Design review of the part built by this model. Coordinates are the model's own, in mm. Give positions to 0.01 mm unless a question says otherwise; leave off trailing zeros. Write each loop counter-clockwise with the first axis right and the second up, starting at its lowest first coordinate (ties: lowest second). Pieces come first, ordered by that corner, then holes. Notation, with made-up numbers: (-3, -5.75) -> (48, -5.75) arc R17 ccw to (48, 21.25) -> close; hole circle Ø10 at (88.25, 19). An arc over 180 degrees is marked (long way). Answer as a JSON object with one key per item and string values.
```python
from build123d import *

# Parameters (mm, degrees)
SKETCH1_W                        = 35
SKETCH1_H                        = 42.3
SKETCH1_W_2                      = 42.3
BOSS_EXTRUDE1_DEPTH              = 2
F_1_8_0_125_DIAMETER_HOLE1_D     = 3.175
F_1_8_0_125_DIAMETER_HOLE1_DEPTH = 4.5
F_1_8_0_125_DIAMETER_HOLE1_TIP   = 0.953866233
SKETCH4_R                        = 11.5
CUT_EXTRUDE1_DEPTH               = 2
CHAMFER1_SIZE                    = 5


with BuildPart() as part:
    # Sketch1 → Boss-Extrude1 (new body)
    with BuildSketch(Plane.XY):
        with Locations((-38.65, 0)):
            Rectangle(SKETCH1_W, SKETCH1_H)
        Rectangle(SKETCH1_W_2, SKETCH1_H)
    extrude(amount=BOSS_EXTRUDE1_DEPTH)

    # 1/8 (0.125) Diameter Hole1
    with Locations(Plane.XY.offset(2)):
        with Locations((-15.5, 15.5), (15.5, 15.5), (15.5, -15.5), (-15.5, -15.5)):
            Hole(F_1_8_0_125_DIAMETER_HOLE1_D / 2, depth=F_1_8_0_125_DIAMETER_HOLE1_DEPTH)
            with Locations((0, 0, -(F_1_8_0_125_DIAMETER_HOLE1_DEPTH + F_1_8_0_125_DIAMETER_HOLE1_TIP / 2))):  # 118° drill point
                Cone(0, F_1_8_0_125_DIAMETER_HOLE1_D / 2, F_1_8_0_125_DIAMETER_HOLE1_TIP, mode=Mode.SUBTRACT)

    # Sketch4 → Cut-Extrude1 (cut)
    with BuildSketch(Plane.XY.offset(2)):
        Circle(SKETCH4_R)
    extrude(amount=-CUT_EXTRUDE1_DEPTH, mode=Mode.SUBTRACT)

    # Chamfer1
    chamfer1_edges = [part.edges().sort_by_distance(p)[0] for p in [
        (21.15, 21.15, 1),
        (21.15, -21.15, 1),
        (-56.15, -21.15, 1),
        (-56.15, 21.15, 1),
    ]]
    chamfer(chamfer1_edges, length=CHAMFER1_SIZE)


solid = part.part
```
(1) We need section D-D, the plane y = -6.5. State the section outline as (x, z) points.
Here are the results:
{"outline": "(-56.15, 0) -> (-9.49, 0) -> (-9.49, 2) -> (-56.15, 2) -> close; (9.49, 0) -> (21.15, 0) -> (21.15, 2) -> (9.49, 2) -> close"}
(2) We need section C-C, the plane x = 0. State the section outline as (y, z) points.
Here are the results:
{"outline": "(-21.15, 0) -> (-11.5, 0) -> (-11.5, 2) -> (-21.15, 2) -> close; (11.5, 0) -> (21.15, 0) -> (21.15, 2) -> (11.5, 2) -> close"}
(3) The part is to be moulded in two halves that separate along Y. For faces 1 (the flat face through (18.7, 18.6, 1)), 2 (the cylindrical face through (-15.16, 13.95, 0.99)), 3 (the flat face through (-18, -21.15, 1)), say which applies: +Y half, -Y half, draft (parallel to the pull), parting line (faces both ways), or undercut.
Here are the results:
{"face 1": "+Y half", "face 2": "undercut", "face 3": "-Y half"}
(4) We need section A-A, the plane z = 1.4. Give the number of separate pieces and of enclosed holes in the cut face, then the cut area to 3 significant figures.
Here are the results:
{"separate pieces": "1", "enclosed holes": "5", "area": "2,770 mm²"}
(5) Clearance check with a flat-ended pin moving along its axis: pin 1 (4 mm diameter, centred on x = -33.5, y = 6, fed in from -Z). State where the tip first meets the part, or that it passes through.
Here are the results:
{"pin 1": "stops at z = 0"}
(6) For line 1 along Y through (x, z) = (15.5, 0.75); line 2 along Y through (x, z) = (0, 0.85); line 3 along X through (y, z) = (-16, 1.1), list the stretches that pass through material, from the lowest coordinate up.
Here are the results:
{"line 1": "y = -21.15 to -17.09, -13.91 to 13.91, 17.09 to 21.15", "line 2": "y = -21.15 to -11.5, 11.5 to 21.15", "line 3": "x = -56.15 to -17.01, -13.99 to 13.99, 17.01 to 21.15"}
(7) We need section B-B, the plane x = -15.5. State the section outline as (y, z) points, then the cut area to 3 significant figures.
Here are the results:
{"outline": "(-21.15, 0) -> (-17.09, 0) -> (-17.09, 2) -> (-21.15, 2) -> close; (-13.91, 0) -> (13.91, 0) -> (13.91, 2) -> (-13.91, 2) -> close; (17.09, 0) -> (21.15, 0) -> (21.15, 2) -> (17.09, 2) -> close", "area": "71.9 mm²"}
